Autodesk Inventor part; units mm, degrees
ref_plane "YZ Plane" through (0, 0, 0) normal (1, 0, 0) x (0, 1, 0)
ref_plane "XZ Plane" through (0, 0, 0) normal (0, 1, 0) x (-1, 0, 0)
ref_plane "XY Plane" through (0, 0, 0) normal (0, 0, 1) x (1, 0, 0)
sketch "Sketch1" plane through (0, 0, 0) normal (0, 1, 0) x (-1, 0, 0)
  line L0 (0, 0) -> (722.517, 0)
  line L1 (722.517, 0) -> (722.517, -100)
  line L2 (722.517, -100) -> (0, -100)
  line L3 (0, -100) -> (0, 0)
  dimension "d0" = 722.517
  dimension "d1" = 100
extrude "Extrusion1" add sketch "Sketch1" along normal blind 50
sketch "Sketch2" plane through (0, 50, 0) normal (0, 1, 0) x (1, 0, 0)
  line L0 (0, 0) -> (0, 100)
  line L1 (-722.517, 100) -> (-722.517, 0)
  line L2 (0, 10) -> (-722.517, 10)
  line L3 (-722.517, 10) -> (-722.517, 90)
  line L4 (-722.517, 90) -> (0, 90)
  line L5 (0, 90) -> (0, 10)
  dimension "d4" = 80
extrude "Extrusion2" cut sketch "Sketch2" against normal blind 40
fillet "Fillet1" radius 4 2 edges at (-361.2585, 10, -90) (-361.2585, 10, -10)
equation "\"BendRadius\" = Thickness"
equation "\"BendReliefWidth\" = Thickness"
equation "\"BendReliefDepth\" = 0.5 * Thickness"
equation "\"CornerReliefSize\" = 4 * Thickness"
equation "\"MinimumRemnant\" = 2 * Thickness"
equation "\"TransitionRadius\" = BendRadius"
equation "\"JacobiRadiusSize\" = BendRadius"
equation "\"GapSize\" = Thickness"
properties part number "Base4"
Geometry: final body of the model. Coordinates: model frame, mm. A direction names the side the tool comes from. Give positions to 0.01 mm unless a question says otherwise; leave off trailing zeros. Write each loop counter-clockwise with the first axis right and the second up, starting at its lowest first coordinate (ties: lowest second). Pieces come first, ordered by that corner, then holes. Notation, with made-up numbers: (62, -26) -> (85, -26) arc R26 cw to (85, 0) -> close; hole circle Ø5 at (-28, -38.75). An arc over 180 degrees is marked (long way). Answer as a JSON object with one key per item and string values.
1. Ray query, probe 1 along Z at (x, y) = (-604, 20.5); probe 2 along Z at (x, y) = (-216, 13); probe 3 along Y at (x, z) = (-53, -41). Return the intervals inside material, ascending. Write a range as from..to.
Ans:
{"probe 1": "z = -100..-90, -10..0", "probe 2": "z = -100..-89.87, -10.13..0", "probe 3": "y = 0..10"}
2. Cut plane A-A on y = 44. Output: boundary loops of the cut face in (x, z).
Ans:
{"outline": "(-722.52, -100) -> (0, -100) -> (0, -90) -> (-722.52, -90) -> close; (-722.52, -10) -> (0, -10) -> (0, 0) -> (-722.52, 0) -> close"}
3. Access query for faces 1 (the flat face through (-356, 32, -10)), 2 (the flat face through (-356, 0, -49)). Directions: +Z, -Z, +X, -X, +Y, -Y. A direction counts if a zero-diameter tool reaches every point of the face in a straight line with its end or side. Return the directions, or none.
Ans:
{"face 1": "+X, -X, +Y", "face 2": "+Z, -Z, +X, -X, -Y"}
4. Cut plane C-C on z = -67.5. Output: boundary loops of the cut face in (x, y).
Ans:
{"outline": "(-722.52, 0) -> (0, 0) -> (0, 10) -> (-722.52, 10) -> close"}
5. Contact query for a flat-ended pin moving along its axis: pin 1 (2 mm diameter, centred on x = -418, z = -34.5, fed in from +Y). Output: stop coordinate, or through.
Ans:
{"pin 1": "stops at y = 10"}
6. Cut plane B-B on x = -450. Output: boundary loops of the cut face in (y, z).
Ans:
{"outline": "(0, -100) -> (50, -100) -> (50, -90) -> (14, -90) arc R4 cw to (10, -86) -> (10, -14) arc R4 cw to (14, -10) -> (50, -10) -> (50, 0) -> (0, 0) -> close"}
7. Mould query, pull axis Z, two halves, no side actions, for faces 3 (the flat face through (0, 8, -51)), 4 (the flat face through (-366, 32, -90)), 5 (the flat face through (-366, 25, -100)). Classes: pulls with the +Z half, pulls with the -Z half, needs draft (parallel to the pull), parting line crosses it, or undercut.
Ans:
{"face 3": "needs draft", "face 4": "undercut", "face 5": "pulls with the -Z half"}
